Check sheet for the modelled part. Datum: model origin and axes. Units: mm. A direction names the side the tool comes from. Give positions to 0.01 mm unless a question says otherwise; leave off trailing zeros. Order: outer loops, then holes, each group sorted by start corner. A loop starts at its lowest first (then second) coordinate and runs counter-clockwise, first axis right, second up.
from build123d import *

# Parameters (mm, degrees)
SKETCH1_R           = 9.525
BOSS_EXTRUDE1_DEPTH = 3.175
CUT_EXTRUDE1_DEPTH  = 0.508


with BuildPart() as part:
    # Sketch1 → Boss-Extrude1 (new body)
    with BuildSketch(Plane(origin=(0, 0, 0), x_dir=(0, 0, -1), z_dir=(1, 0, 0))):
        Circle(SKETCH1_R)
        Polygon((7.772289324, 0), (3.886144662, 6.731), (-3.886144662, 6.731), (-7.772289324, 0), (-3.886144662, -6.731), (3.886144662, -6.731), align=None, mode=Mode.SUBTRACT)
    extrude(amount=BOSS_EXTRUDE1_DEPTH)

    # Sketch2 → Cut-Extrude1 (cut)
    with BuildSketch(Plane(origin=(3.175, 0, 0), x_dir=(0, 0, -1), z_dir=(1, 0, 0))):
        Polygon((-2.112938805, 10.442477423), (-1.465803389, 10.442477423), (-1.465803389, 6.942477423), (-1.779905953, 6.942477423), (-1.779905953, 10.083503064), (-2.318367491, 10.083503064), align=None)
        Polygon((0.579368887, 10.442477423), (1.226504304, 10.442477423), (1.226504304, 6.942477423), (0.91240174, 6.942477423), (0.91240174, 10.083503064), (0.373940201, 10.083503064), align=None)
    extrude(amount=-CUT_EXTRUDE1_DEPTH, mode=Mode.SUBTRACT)


solid = part.part
1) Depth check by flat-ended pin: pin 1 Ø1 at (x, y) = (2.5, -5) entering from -Z (3 decimals); pin 2 Ø0.6 at (x, y) = (3, 7.5) entering from +Z; pin 3 Ø0.6 at (x, y) = (3, 8) entering from +Z. Enter the tip coordinate at first touch or a pass-through.
Recorded:
pin 1: stops at z = -8.395
pin 2: stops at z = 6.24
pin 3: stops at z = 5.61
2) Draft check along Y on faces 1 (the face through (1.565, -5.796, 7.559)), 2 (the face through (0, -2.8, 6.4)), 3 (the face through (2, 6.731, 0)), 4 (the face through (2, -6.731, 0)). Enter one of: +Y half, -Y half, draft (parallel to the pull), parting line (faces both ways), or undercut.
Recorded:
face 1: parting line
face 2: draft
face 3: undercut
face 4: undercut
3) Section check D-D, the plane y = -7. Record the cut outline in (x, z) (3 decimals), then the cut area to 3 significant figures.
Recorded:
outline: (0, -6.46) - (3.175, -6.46) - (3.175, 6.46) - (0, 6.46) - close
area: 41.0 mm2
4) Section check A-A, the plane z = 0. Record the cut outline in (x, y) (3 decimals).
Recorded:
outline: (0, -9.525) - (3.175, -9.525) - (3.175, -6.731) - (0, -6.731) - close; (0, 6.731) - (3.175, 6.731) - (3.175, 9.525) - (0, 9.525) - close
5) Section check C-C, the plane x = 1.15. Record the cut outline in (y, z) (3 decimals), then the cut area to 3 significant figures.
Recorded:
outline: circle Ø19.05 at (0, 0); hole (-6.731, -3.886) - (0, -7.772) - (6.731, -3.886) - (6.731, 3.886) - (0, 7.772) - (-6.731, 3.886) - close
area: 128 mm2
6) Material ranges on L1, parallel to Z at x = 0.4, y = -4; L2, parallel to Y at x = 1.75, z = -0.5; L3, parallel to Y at x = 0.75, z = -4.25, recorded low to high.
Recorded:
L1: z = -8.64 to -5.46, 5.46 to 8.64
L2: y = -9.51 to -6.73, 6.73 to 9.51
L3: y = -8.52 to -6.1, 6.1 to 8.52
7) Section check B-B, the plane y = -1. Record the cut outline in (x, z) (3 decimals), then the cut area to 3 significant figures.
Recorded:
outline: (0, -9.472) - (3.175, -9.472) - (3.175, -7.195) - (0, -7.195) - close; (0, 7.195) - (3.175, 7.195) - (3.175, 9.472) - (0, 9.472) - close
area: 14.5 mm2
8) Set-up check for faces 5 (the face through (3.175, -2.8, 6.4)), 6 (the face through (1.565, 3.318, -5.856)): record each of +Z, -Z, +X, -X, +Y, -Y from which the full face is reachable in a straight line by a thin tool's end or side.
Recorded:
face 5: +Z, -Z, +X, +Y, -Y
face 6: +X, -X
